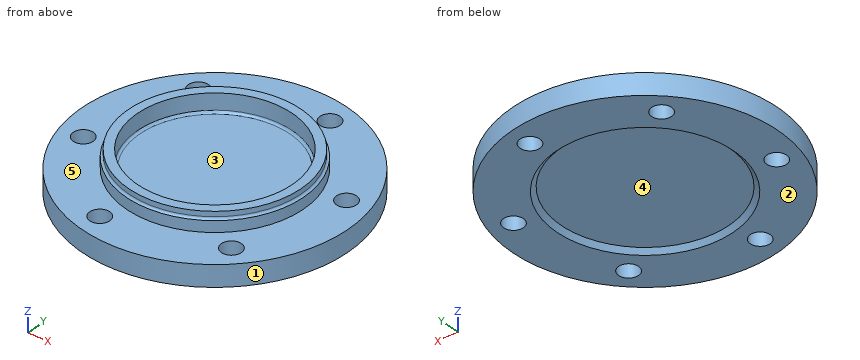
from build123d import *

# Parameters (mm, degrees)
M8_CLEARANCE_HOLE1_D = 9
CIRPATTERN1_COUNT    = 6


with BuildPart() as part:
    # Sketch1 → Revolve1 (revolve)
    with BuildSketch(Plane(origin=(0, 0, 0), x_dir=(0, 0, -1), z_dir=(1, 0, 0))):
        with BuildLine():
            Line((0, 0), (0, 34))
            ThreePointArc((0, 34), (-0.292893219, 34.707106781), (-1, 35))
            Line((-1, 35), (-8.25, 35))
            Line((-8.25, 35), (-8.25, 39))
            Line((-8.25, 39), (-6, 39))
            ThreePointArc((-6, 39), (-5.292893219, 39.292893219), (-5, 40))
            Line((-5, 40), (0, 40))
            Line((0, 40), (0, 60))
            Line((0, 60), (9.6, 60))
            Line((9.6, 60), (9.6, 40))
            Line((9.6, 40), (7.6, 38))
            Line((7.6, 38), (7.6, 0))
            Line((7.6, 0), (0, 0))
        make_face()
    revolve(axis=Axis((0, 0, -9.6), (0, 0, 1)))

    # M8 Clearance Hole1 (through all)
    with Locations(Plane(origin=(0, 0, -9.6), x_dir=(-1, 0, 0), z_dir=(0, 0, -1))):
        with Locations((35.355339059, 35.355339059)):
            m8_clearance_hole1 = Hole(M8_CLEARANCE_HOLE1_D / 2)

    # CirPattern1: M8 Clearance Hole1 ×6 about axis
    cirpattern1_axis = Axis((0, 0, 0), (0, 0, 1))
    for i in range(1, CIRPATTERN1_COUNT):
        add(m8_clearance_hole1.rotate(cirpattern1_axis, i * 360 / CIRPATTERN1_COUNT), mode=Mode.SUBTRACT)


solid = part.part
Design review of the part built by this model. Coordinates are the model's own, in mm. Face numbers are marked on the shaded views. A direction names the side the tool comes from. Coordinates: 2 decimals unless noted, no trailing zeros. Write each loop counter-clockwise with the first axis right and the second up, starting at its lowest first coordinate (ties: lowest second). Pieces come first, ordered by that corner, then holes. Notation, with made-up numbers: (77.5, 27) -> (101.5, 27) arc R7 cw to (101.5, 31) -> close; hole circle Ø6 at (54, 14). An arc over 180 degrees is marked (long way). Write each question's results on one line, items separated by ' | '. Start each with the question number.
(1) Clearance check with flat-ended pins moving along their axes: P1, Ø8, axis at x = 12, y = 8, coming from the +Z side; P2, Ø2, axis at x = 30, y = 10, coming from the -Z side; P3, Ø8, axis at x = -43, z = -6.5, coming from the -Y side; P4, Ø5.5, axis at x = 35.36, y = -35.36, coming from the -Z side. State where each tip first meets the part, or that it passes through.
(2) Take a section at A-A on x = 49. Write out the cut boundary in (y, z), and give its area (3 significant figures).
(3) Tool access review of the marked faces 4 and 5: name each direction out of +Z, -Z, +X, -X, +Y, -Y from which nothing blocks a thin tool from reaching the whole face with its end or side.
(4) Take a section at B-B on y = 47.5. Write out the cut boundary in (x, z), and give its area (3 significant figures).
(5) Take a section at C-C on z = -5.5. Write out the cut boundary in (x, y).
(6) For line 1 along Y through (x, z) = (0, 3.75); line 2 along X through (y, z) = (0, 6.75); line 3 along X through (y, z) = (-51.5, -4.75), list the stretches that pass through material, from the lowest coordinate up. Write a range as from..to.
(7) Take a section at D-D on x = 0. Write out the cut boundary in (y, z).
(8) The part is to be moulded in two halves that separate along Y. For the marked faces 1, 2 and 3, say which applies: pulls with the +Y half, pulls with the -Y half, needs draft (parallel to the pull), parting line crosses it, or undercut.
Results found:
1) P1: stops at z = 0 | P2: stops at z = -7.6 | P3: stops at y = -45.6 | P4: passes through
2) outline: (-34.63, -9.6) -> (8.5, -9.6) -> (8.5, 0) -> (-34.63, 0) -> close; (17.39, -9.6) -> (34.63, -9.6) -> (34.63, 0) -> (17.39, 0) -> close | area: 579 mm2
3) face 4: -Z | face 5: +Z
4) outline: (-36.66, -9.6) -> (8.51, -9.6) -> (8.51, 0) -> (-36.66, 0) -> close; (17.37, -9.6) -> (36.66, -9.6) -> (36.66, 0) -> (17.37, 0) -> close | area: 619 mm2
5) outline: circle Ø120 at (0, 0); hole circle Ø9 at (-48.3, -12.94); hole circle Ø9 at (-35.36, 35.36); hole circle Ø9 at (-12.94, -48.3); hole circle Ø9 at (12.94, 48.3); hole circle Ø9 at (35.36, -35.36); hole circle Ø9 at (48.3, 12.94)
6) line 1: y = -40..-35, 35..40 | line 2: x = -39..-35, 35..39 | line 3: x = -30.79..-16.1, -9.78..30.79
7) outline: (-60, -9.6) -> (-40, -9.6) -> (-38, -7.6) -> (38, -7.6) -> (40, -9.6) -> (60, -9.6) -> (60, 0) -> (40, 0) -> (40, 5) arc R1 cw to (39, 6) -> (39, 8.25) -> (35, 8.25) -> (35, 1) arc R1 cw to (34, 0) -> (-34, 0) arc R1 cw to (-35, 1) -> (-35, 8.25) -> (-39, 8.25) -> (-39, 6) arc R1 cw to (-40, 5) -> (-40, 0) -> (-60, 0) -> close
8) face 1: parting line crosses it | face 2: needs draft | face 3: undercut
